The listing builds one solid part. Answer for the finished solid, in the listing's coordinates (mm). A direction names the side the tool comes from. Coordinates: 2 decimals unless noted, no trailing zeros. Order: outer loops, then holes, each group sorted by start corner. A loop starts at its lowest first (then second) coordinate and runs counter-clockwise, first axis right, second up. Notation, with made-up numbers: (4.25, 72.5) - (51.25, 72.5) arc R28 cw to (51.25, 106.5) - close; hole circle Ø2 at (78.25, 71). An arc over 180 degrees is marked (long way). Use a Markdown table: item, result. Add a question column.
Item 1: The mould has two halves that part along Y. Classify faces 1 (the flat face through (1.479, 41.295, 20.766)), 2 (the flat face through (1, 2.5, -25)), 3 (the cylindrical face through (1.52, 7.32, -29.63)), 4 (the flat face through (1, 5, 30)): released by +Y, released by -Y, zero draft, split by the parting line, or undercut.
Item 2: For faces 5 (the flat face through (1, 2.5, 25)), 6 (the flat face through (1.48, 26.03, 35.2)), 7 (the flat face through (1, 0, -20)), 8 (the flat face through (1, 2.5, 0)), determine the directions among +Z, -Z, +X, -X, +Y, -Y from which every point of the face is accessible in a straight line to the end or side of a thin tool.
Item 3: Flat-ended cylindrical pins translate along their axes: P1, Ø5, axis at y = 52.93, z = 23.91, coming from the +X side; P2, Ø1.5, axis at x = 1.5, z = 40.5, coming from the +Y side; P3, Ø1, axis at x = 0.5, z = 8, coming from the +Y side; P4, Ø0.9, axis at x = 1.5, y = 0, coming from the +Z side. Find the tip coordinate at first contact, or state that the pin passes through.
Item 4: The part is cut by section C-C, the plane x = 1.3. Give the vertices of the cut face in (y, z).
Item 5: The part is cut by section A-A, the plane z = 39. Give the vertices of the cut face in (x, y).
Item 6: The part is cut by section B-B, the plane y = 36. Give the vertices of the cut face in (x, z).
Item 7: Find the intervals of material crossed by line 1 along Z through (x, y) = (1.85, 54); line 2 along Z through (x, y) = (0.85, 8); line 3 along Y through (x, z) = (2.5, -7.5), in increasing order.
from build123d import *

# Parameters (mm, degrees)
BOSS_EXTRUDE1_DEPTH = 3
CUT_EXTRUDE2_DEPTH  = 10
SKETCH5_R           = 1.5
CUT_EXTRUDE3_DEPTH  = 10
FILLET1_R           = 10
FILLET2_R           = 1
FILLET3_R           = 5


with BuildPart() as part:
    # Sketch3 → Boss-Extrude1 (new body)
    with BuildSketch(Plane(origin=(0, 0, 0), x_dir=(0, 0, -1), z_dir=(1, 0, 0))):
        with BuildLine():
            Line((15, -2.5), (20, -2.5))
            Line((20, -2.5), (20, 2.5))
            Line((20, 2.5), (30, 2.5))
            Line((30, 2.5), (30, 7.5))
            Line((30, 7.5), (-19.497474683, 56.997474683))
            ThreePointArc((-19.497474683, 56.997474683), (-56.194666741, 49.697949335), (-35.40737726, 18.587572106))
            Line((-35.40737726, 18.587572106), (-30, 7.5))
            Line((-30, 7.5), (-30, 2.5))
            Line((-30, 2.5), (-20, 2.5))
            Line((-20, 2.5), (-20, -2.5))
            Line((-20, -2.5), (-15, -2.5))
            Line((-15, -2.5), (-15, 2.5))
            Line((-15, 2.5), (15, 2.5))
            Line((15, 2.5), (15, -2.5))
        make_face()
    extrude(amount=BOSS_EXTRUDE1_DEPTH)

    # Sketch4 → Cut-Extrude2 (cut)
    with BuildSketch(Plane.ZY):
        Polygon((35.372021921, 55.901459172), (5.744247789, 26.273685041), (20.593490194, 11.424442636), (50.221264326, 41.052216767), align=None)
    extrude(amount=-CUT_EXTRUDE2_DEPTH, mode=Mode.SUBTRACT)

    # Sketch5 → Cut-Extrude3 (cut)
    with BuildSketch(Plane.ZY):
        with Locations((22.471283385, 7.5)):
            Circle(SKETCH5_R)
        with Locations((-22.528716615, 7.5)):
            Circle(SKETCH5_R)
        with Locations((23.910377597, 52.925096223)):
            Circle(SKETCH5_R)
        with Locations((47.244901376, 29.590572444)):
            Circle(SKETCH5_R)
    extrude(amount=-CUT_EXTRUDE3_DEPTH, mode=Mode.SUBTRACT)

    # Fillet1
    fillet1_edges = [part.edges().sort_by_distance(p)[0] for p in [
        (1.5, 18.587572106, 35.40737726),
    ]]
    fillet(fillet1_edges, radius=FILLET1_R)

    # Fillet2
    fillet2_edges = [part.edges().sort_by_distance(p)[0] for p in [
        (1.5, -2.5, -20),
        (1.5, -2.5, -15),
        (1.5, -2.5, 15),
        (1.5, -2.5, 20),
    ]]
    fillet(fillet2_edges, radius=FILLET2_R)

    # Fillet3
    fillet3_edges = [part.edges().sort_by_distance(p)[0] for p in [
        (1.5, 7.5, -30),
    ]]
    fillet(fillet3_edges, radius=FILLET3_R)


solid = part.part
Solution:
| question | item | result |
|---|---|---|
| 1 | face 1 | undercut |
| 1 | face 2 | released by -Y |
| 1 | face 3 | released by +Y |
| 1 | face 4 | zero draft |
| 2 | face 5 | +Z, +X, -X, -Y |
| 2 | face 6 | +X, -X |
| 2 | face 7 | -Z, +X, -X, -Y |
| 2 | face 8 | +X, -X, -Y |
| 3 | P1 | stops at x = 3 |
| 3 | P2 | stops at y = 63.16 |
| 3 | P3 | stops at y = 46 |
| 3 | P4 | stops at z = 20 |
| 4 | outline | (-2.5, -19) arc R1 ccw to (-1.5, -20) - (2.5, -20) - (2.5, -30) - (5.43, -30) arc R5 ccw to (8.96, -28.54) - (57, 19.5) arc R22.5 ccw (long way) to (19.05, 39.96) arc R10 cw to (13.64, 33) - (7.5, 30) - (2.5, 30) - (2.5, 20) - (-1.5, 20) arc R1 ccw to (-2.5, 19) - (-2.5, 16) arc R1 ccw to (-1.5, 15) - (2.5, 15) - (2.5, -15) - (-1.5, -15) arc R1 ccw to (-2.5, -16) - close; hole circle Ø3 at (7.5, -22.53); hole circle Ø3 at (7.5, 22.47); hole (11.42, 20.59) - (26.27, 5.74) - (55.9, 35.37) - (41.05, 50.22) - close; hole circle Ø3 at (29.59, 47.24); hole circle Ø3 at (52.93, 23.91) |
| 5 | outline | (0, 18.8) - (3, 18.8) - (3, 29.83) - (0, 29.83) - close; (0, 52.27) - (3, 52.27) - (3, 63.3) - (0, 63.3) - close |
| 6 | outline | (0, -1.5) - (3, -1.5) - (3, 15.47) - (0, 15.47) - close; (0, 45.17) - (3, 45.17) - (3, 57.32) - (0, 57.32) - close |
| 7 | line 1 | z = 16.5 to 22.86, 24.96 to 33.47, 37.27 to 53.83 |
| 7 | line 2 | z = -29.29 to -23.94, -21.11 to 21.06, 23.89 to 30.24 |
| 7 | line 3 | y = 2.5 to 30 |
